Here's how the part is built. I have some questions about the finished solid (model axes, mm). Face numbers are marked on the shaded views. A direction names the side the tool comes from. Round coordinates to 2 decimals unless told otherwise and drop trailing zeros. Write each loop counter-clockwise with the first axis right and the second up, starting at its lowest first coordinate (ties: lowest second). Pieces come first, ordered by that corner, then holes. Notation, with made-up numbers: (68.25, 84) -> (109.25, 84) arc R17 ccw to (109.25, 88) -> close; hole circle Ø10 at (29.25, -12). An arc over 180 degrees is marked (long way). Put each result on its own line as item: value. Start each with the question number.
1. Suppose I cut it at B-B (x = -18.5). Please give me the cut outline in (y, z) (3 decimals).
2. Which directions (+Z, -Z, +X, -X, +Y, -Y) give clear straight access to the entire face, cutting with the end or side of a thin tool? Please do the marked faces 4, 5 and 6.
3. For pin 1 (9.5 mm diameter, centred on x = 5.5, z = 30.5, fed in from -Y); pin 2 (8 mm diameter, centred on x = -4.5, y = -10, fed in from +Z); pin 3 (1.5 mm diameter, centred on x = -11.5, z = 8, fed in from +Y), each with a flat end and sliding along its axis, tell me the tip position at first contact or that it passes through.
4. Suppose I cut it at C-C (y = 32.5). Please give me the cut outline in (x, z), then the cut area to 3 significant figures.
5. Suppose I cut it at D-D (z = 15). Please give me the cut outline in (x, y), then the cut area to 3 significant figures.
6. I need wall thicknesses on probe 1 along X at (y, z) = (20.5, 21.5); probe 2 along Y at (x, z) = (9, 29); probe 3 along Z at (x, y) = (4, 12.5). Which ranges of each line are inside material? Lowest first, please. Write a range as from..to.
7. We'd pull the mould along Y, two halves only. Please class the marked faces 1, 2 and 3: +Y half, -Y half, draft (parallel to the pull), parting line (faces both ways), or undercut.
8. Suppose I cut it at A-A (y = -5). Please give me the cut outline in (x, z), then the cut area to 3 significant figures.
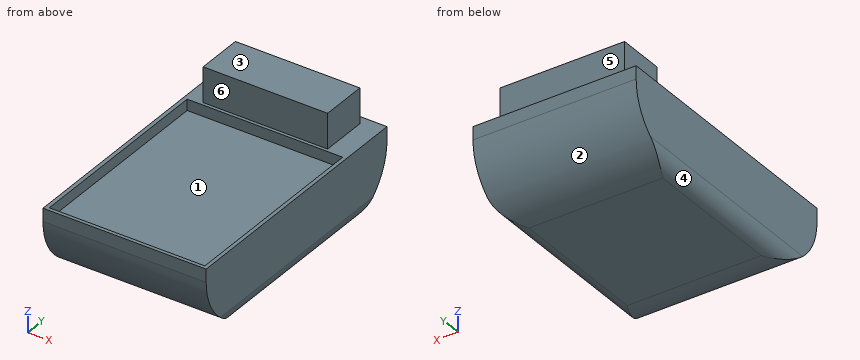
```python
from build123d import *

# Parameters (mm, degrees)
F0_W        = 55.9
F0_H        = 90
F1_DEPTH    = 25
F2_R        = 20.5208152802
F3_W        = 53.3
F3_H        = 68.6
F4_DEPTH    = 3.8
F5_T1_DEPTH = 91.4583694397
F6_T1_DEPTH = 91.4583694397
F8_DEPTH    = 12


# Not quite as in the source:
# - a fillet or chamfer that OpenCascade refuses, or shapes differently, is made with other operations: its cross-section is extruded or revolved along the edge and cut away or added


with BuildPart() as f1:
    # F0 (on Top) → F1 (new body)
    with BuildSketch(Plane.XY):
        with Locations((2.1647780098, -0.8441807004)):
            Rectangle(F0_W, F0_H)
    extrude(amount=F1_DEPTH)

    # F2
    f2_edges = [f1.edges().sort_by_distance(p)[0] for p in [
        (2.164778, -45.844181, 0),
        (2.164778, 44.155819, 0),
    ]]
    fillet(f2_edges, radius=F2_R)

    # F3 (on face) → F4 (cut)
    with BuildSketch(Plane.XY.offset(25)):
        with Locations((2.2094916642, -10.3566651821)):
            Rectangle(F3_W, F3_H)
    extrude(amount=-F4_DEPTH, mode=Mode.SUBTRACT)

    # F5: fillet of radius 5 on 1 edges, made by hand

    # F5_s2 → F5_t1 (cut)
    with BuildSketch(Plane.XZ.offset(-44.8850040195)):
        with BuildLine():
            ThreePointArc((25.1147780098, 0), (28.6503119157, 1.4644660941), (30.1147780098, 5))
            Line((30.1147780098, 5), (30.1147780098, 0))
            Line((30.1147780098, 0), (25.1147780098, 0))
        make_face()
    extrude(amount=F5_T1_DEPTH, mode=Mode.SUBTRACT)

    # F6: fillet of radius 5 on 1 edges, made by hand

    # F6_s2 → F6_t1 (cut)
    with BuildSketch(Plane.XZ.offset(-44.8850040195)):
        with BuildLine():
            ThreePointArc((-25.7852219902, 5), (-24.3207558961, 1.4644660941), (-20.7852219902, 0))
            Line((-20.7852219902, 0), (-25.7852219902, 0))
            Line((-25.7852219902, 0), (-25.7852219902, 5))
        make_face()
    extrude(amount=F6_T1_DEPTH, mode=Mode.SUBTRACT)

    # F7 (on face) → F8 (join)
    with BuildSketch(Plane.XY.offset(25)):
        Polygon((22.9460150003, 41.0868413746), (-19.7153221816, 41.0868413746), (-19.7153221816, 25.0466242433), (22.930214506, 25.0466242433), align=None)
    extrude(amount=F8_DEPTH)


solid = f1.part
```
Verdict:
1. outline: (-45.844, 20.521) arc R20.521 ccw to (-25.323, 0) -> (23.635, 0) arc R20.521 ccw to (44.156, 20.521) -> (44.156, 25) -> (41.087, 25) -> (41.087, 37) -> (25.047, 37) -> (25.047, 25) -> (23.943, 25) -> (23.943, 21.2) -> (-44.657, 21.2) -> (-44.657, 25) -> (-45.844, 25) -> close
2. face 4: -Z, -X, +Y, -Y
2. face 5: +Z, +X, -X, +Y
2. face 6: +Z, +X, -X, -Y
3. pin 1: stops at y = 25.05
3. pin 2: stops at z = 21.2
3. pin 3: stops at y = 40.44
4. outline: (-25.79, 5) arc R5 ccw to (-24.8, 2.01) -> (29.12, 2.01) arc R5 ccw to (30.11, 5) -> (30.11, 25) -> (22.94, 25) -> (22.94, 37) -> (-19.72, 37) -> (-19.72, 25) -> (-25.79, 25) -> close
4. area: 1,790 mm^2
5. outline: (-25.79, -45.09) -> (30.11, -45.09) -> (30.11, 43.4) -> (-25.79, 43.4) -> close
5. area: 4,950 mm^2
6. probe 1: x = -25.79..-24.44, 28.86..30.11
6. probe 2: y = 25.05..41.09
6. probe 3: z = 0..21.2
7. face 1: undercut
7. face 2: +Y half
7. face 3: draft
8. outline: (-25.79, 5) arc R5 ccw to (-20.79, 0) -> (25.11, 0) arc R5 ccw to (30.11, 5) -> (30.11, 25) -> (28.86, 25) -> (28.86, 21.2) -> (-24.44, 21.2) -> (-24.44, 25) -> (-25.79, 25) -> close
8. area: 1,180 mm^2
